Work out the finished part from the listing and answer in its coordinate system (mm). Round coordinates to 2 decimals unless told otherwise and drop trailing zeros. Write each loop counter-clockwise with the first axis right and the second up, starting at its lowest first coordinate (ties: lowest second). Pieces come first, ordered by that corner, then holes. Notation, with made-up numbers: (11, 6) - (22, 6) arc R13 cw to (22, 28) - close; hole circle Ø2 at (55, 89). An arc over 180 degrees is marked (long way). Answer as a JSON object with one key per item and string values.
```python
from build123d import *

# Parameters (mm, degrees)
SKETCH1_W           = 53.2
SKETCH1_H           = 101.6
SKETCH1_R           = 1.25
BOSS_EXTRUDE1_DEPTH = 6.35


with BuildPart() as part:
    # Sketch1 → Boss-Extrude1 (new body)
    with BuildSketch(Plane(origin=(0, 0, 0), x_dir=(1, 0, 0), z_dir=(0, 1, 0))):
        with Locations((-26.6, 50.8)):
            Rectangle(SKETCH1_W, SKETCH1_H)
        with Locations((-50.7, 88.9)):
            Circle(SKETCH1_R, mode=Mode.SUBTRACT)
        with Locations((-2.5, 95.05)):
            Circle(SKETCH1_R, mode=Mode.SUBTRACT)
        with Locations((-35.5, 64.8)):
            Circle(SKETCH1_R, mode=Mode.SUBTRACT)
        with Locations((-7.6, 64.8)):
            Circle(SKETCH1_R, mode=Mode.SUBTRACT)
        with Locations((-50.7, 14)):
            Circle(SKETCH1_R, mode=Mode.SUBTRACT)
        with Locations((-2.5, 12.7)):
            Circle(SKETCH1_R, mode=Mode.SUBTRACT)
    extrude(amount=BOSS_EXTRUDE1_DEPTH)


solid = part.part
```
Item 1: A cutting plane is placed at D-D (x = -35.5). Write down the section's boundary in (y, z).
Results found:
{"outline": "(0, -101.6) - (6.35, -101.6) - (6.35, -66.05) - (0, -66.05) - close; (0, -63.55) - (6.35, -63.55) - (6.35, 0) - (0, 0) - close"}
Item 2: A cutting plane is placed at A-A (x = -50.7). Write down the section's boundary in (y, z), and give its area (3 significant figures).
Results found:
{"outline": "(0, -101.6) - (6.35, -101.6) - (6.35, -90.15) - (0, -90.15) - close; (0, -87.65) - (6.35, -87.65) - (6.35, -15.25) - (0, -15.25) - close; (0, -12.75) - (6.35, -12.75) - (6.35, 0) - (0, 0) - close", "area": "613 mm²"}
Item 3: Determine the mould class of faces 1 (the flat face through (-27, 3, -101.6)), 2 (the flat face through (-53.2, 3, -50)), 3 (the cylindrical face through (-1.923, 3.131, -93.941)) for opening direction X: pulls with the +X half, pulls with the -X half, needs draft (parallel to the pull), parting line crosses it, or undercut.
Results found:
{"face 1": "needs draft", "face 2": "pulls with the -X half", "face 3": "undercut"}
Item 4: A cutting plane is placed at B-B (z = -64.8). Write down the section's boundary in (x, y), and give its area (3 significant figures).
Results found:
{"outline": "(-53.2, 0) - (-36.75, 0) - (-36.75, 6.35) - (-53.2, 6.35) - close; (-34.25, 0) - (-8.85, 0) - (-8.85, 6.35) - (-34.25, 6.35) - close; (-6.35, 0) - (0, 0) - (0, 6.35) - (-6.35, 6.35) - close", "area": "306 mm²"}
Item 5: Consider line 1 along Z through (x, y) = (-2.5, 3.5); line 2 along X through (y, z) = (2.5, -64.8); line 3 along Z through (x, y) = (-50.7, 2.75). Determine where each line is inside the solid, lowest interval first.
Results found:
{"line 1": "-101.6 to -96.3, -93.8 to -13.95, -11.45 to 0", "line 2": "-53.2 to -36.75, -34.25 to -8.85, -6.35 to 0", "line 3": "-101.6 to -90.15, -87.65 to -15.25, -12.75 to 0"}
Item 6: A cutting plane is placed at C-C (z = -88.9). Write down the section's boundary in (x, y), and give its area (3 significant figures).
Results found:
{"outline": "(-53.2, 0) - (-51.95, 0) - (-51.95, 6.35) - (-53.2, 6.35) - close; (-49.45, 0) - (0, 0) - (0, 6.35) - (-49.45, 6.35) - close", "area": "322 mm²"}
